The listing builds one solid part. Answer for the finished solid, in the listing's coordinates (mm). A direction names the side the tool comes from. Round coordinates to 2 decimals unless told otherwise and drop trailing zeros. Write each loop counter-clockwise with the first axis right and the second up, starting at its lowest first coordinate (ties: lowest second). Pieces come first, ordered by that corner, then holes.
(1) A cutting plane is placed at D-D, the plane z = -68. Give the vertices of the cut face in (x, y), and give its area (3 significant figures).
(2) A cutting plane is placed at B-B, the plane y = -5.5. Give the vertices of the cut face in (x, z), and give its area (3 significant figures).
(3) For faces 1 (the face through (0, 0, 0)), 2 (the face through (5, 12, -6.35)), 3 (the face through (-5.506, -24.796, -3.131)), determine the directions among +Z, -Z, +X, -X, +Y, -Y from which every point of the face is accessible in a straight line to the end or side of a thin tool.
(4) A cutting plane is placed at A-A, the plane x = 22. Give the vertices of the cut face in (y, z).
(5) Each of these flat-tipped pins is pushed along its axis until it touches: pin 1 Ø1.5 at (x, z) = (-12, -14) entering from -Y; pin 2 Ø1.5 at (y, z) = (-5.5, -45.5) entering from -X; pin 3 Ø1 at (x, z) = (7, -29.5) entering from -Y. Where does it stop, or does it pass through?
(6) Find the intervals of material crossed by probe 1 along Z at (x, y) = (-2.5, -12.5); probe 2 along Z at (x, y) = (-15.5, -40.5); probe 3 along X at (y, z) = (8, -9), in increasing order.
(7) A cutting plane is placed at C-C, the plane x = 0. Give the vertices of the cut face in (y, z).
from build123d import *

# Parameters (mm, degrees)
F0_R     = 25.4
F1_DEPTH = 6.35
F2_R     = 12.7
F3_DEPTH = 88.9
F4_W     = 139.7
F4_H     = 101.6
F5_DEPTH = 8.89


with BuildPart() as f1:
    # F0 (on Top) → F1 (new body)
    with BuildSketch(Plane.XY):
        Circle(F0_R)
    extrude(amount=-F1_DEPTH)

    # F2 (on face) → F3 (join)
    with BuildSketch(Plane(origin=(0, 0, -6.35), x_dir=(1, 0, 0), z_dir=(0, 0, -1))):
        Circle(F2_R)
    extrude(amount=F3_DEPTH)

    # F4 (on face) → F5 (join)
    with BuildSketch(Plane(origin=(0, 0, -95.25), x_dir=(1, 0, 0), z_dir=(0, 0, -1))):
        Rectangle(F4_W, F4_H)
    extrude(amount=F5_DEPTH)


solid = f1.part
Solutions:
1. outline: circle Ø25.4 at (0, 0)
1. area: 507 mm2
2. outline: (-69.85, -104.14) - (69.85, -104.14) - (69.85, -95.25) - (11.45, -95.25) - (11.45, -6.35) - (24.8, -6.35) - (24.8, 0) - (-24.8, 0) - (-24.8, -6.35) - (-11.45, -6.35) - (-11.45, -95.25) - (-69.85, -95.25) - close
2. area: 3,590 mm2
3. face 1: +Z, +X, -X, +Y, -Y
3. face 2: none
3. face 3: +Z
4. outline: (-50.8, -104.14) - (50.8, -104.14) - (50.8, -95.25) - (-50.8, -95.25) - close; (-12.69, -6.35) - (12.69, -6.35) - (12.69, 0) - (-12.69, 0) - close
5. pin 1: stops at y = -5.89
5. pin 2: stops at x = -11.78
5. pin 3: stops at y = -10.91
6. probe 1: z = -104.14 to -95.25, -6.35 to 0
6. probe 2: z = -104.14 to -95.25
6. probe 3: x = -9.86 to 9.86
7. outline: (-50.8, -104.14) - (50.8, -104.14) - (50.8, -95.25) - (12.7, -95.25) - (12.7, -6.35) - (25.4, -6.35) - (25.4, 0) - (-25.4, 0) - (-25.4, -6.35) - (-12.7, -6.35) - (-12.7, -95.25) - (-50.8, -95.25) - close
